Part model, mm, in its own coordinate system. Face numbers are marked on the shaded views. A direction names the side the tool comes from. Coordinates: 2 decimals unless noted, no trailing zeros. Order: outer loops, then holes, each group sorted by start corner. A loop starts at its lowest first (then second) coordinate and runs counter-clockwise, first axis right, second up.
```python
from build123d import *

# Parameters (mm, degrees)
SKETCH_1_R          = 11
EXTRUDE_1_DEPTH     = 2
SKETCH_2_R          = 5
EXTRUDE_2_DEPTH     = 10
SKETCH_4_R          = 3
CUT_EXTRUDE_2_DEPTH = 13
CUT_EXTRUDE_3_REACH = 4
SKETCH_5_R          = 1.5


with BuildPart() as part:
    # 草图1 → 凸台-拉伸1 (new body)
    with BuildSketch(Plane.XY):
        Circle(SKETCH_1_R)
    extrude(amount=EXTRUDE_1_DEPTH)

    # 草图2 → 凸台-拉伸2 (add)
    with BuildSketch(Plane.XY.offset(2)):
        Circle(SKETCH_2_R)
    extrude(amount=EXTRUDE_2_DEPTH)

    # 草图4 → 切除-拉伸2 (cut, through all)
    with BuildSketch(Plane.XY.offset(12)):
        Circle(SKETCH_4_R)
    extrude(amount=-CUT_EXTRUDE_2_DEPTH, mode=Mode.SUBTRACT)

    # 草图5 → 切除-拉伸3 (cut, up to next)
    with BuildSketch(Plane.XY.offset(2), mode=Mode.PRIVATE) as cut_extrude_3_sk1:
        with Locations((-8, 0)):
            Circle(SKETCH_5_R)
    cut_extrude_3_tool1 = extrude(cut_extrude_3_sk1.sketch, amount=-CUT_EXTRUDE_3_REACH, mode=Mode.PRIVATE) & part.part
    add(cut_extrude_3_tool1.solids().sort_by_distance((-8, 0, 2))[0], mode=Mode.SUBTRACT)
    # 草图5 → 切除-拉伸3 (cut, up to next)
    with BuildSketch(Plane.XY.offset(2), mode=Mode.PRIVATE) as cut_extrude_3_sk2:
        with Locations((0, 8)):
            Circle(SKETCH_5_R)
    cut_extrude_3_tool2 = extrude(cut_extrude_3_sk2.sketch, amount=-CUT_EXTRUDE_3_REACH, mode=Mode.PRIVATE) & part.part
    add(cut_extrude_3_tool2.solids().sort_by_distance((0, 8, 2))[0], mode=Mode.SUBTRACT)
    # 草图5 → 切除-拉伸3 (cut, up to next)
    with BuildSketch(Plane.XY.offset(2), mode=Mode.PRIVATE) as cut_extrude_3_sk3:
        with Locations((8, 0)):
            Circle(SKETCH_5_R)
    cut_extrude_3_tool3 = extrude(cut_extrude_3_sk3.sketch, amount=-CUT_EXTRUDE_3_REACH, mode=Mode.PRIVATE) & part.part
    add(cut_extrude_3_tool3.solids().sort_by_distance((8, 0, 2))[0], mode=Mode.SUBTRACT)
    # 草图5 → 切除-拉伸3 (cut, up to next)
    with BuildSketch(Plane.XY.offset(2), mode=Mode.PRIVATE) as cut_extrude_3_sk4:
        with Locations((0, -8)):
            Circle(SKETCH_5_R)
    cut_extrude_3_tool4 = extrude(cut_extrude_3_sk4.sketch, amount=-CUT_EXTRUDE_3_REACH, mode=Mode.PRIVATE) & part.part
    add(cut_extrude_3_tool4.solids().sort_by_distance((0, -8, 2))[0], mode=Mode.SUBTRACT)


solid = part.part
```
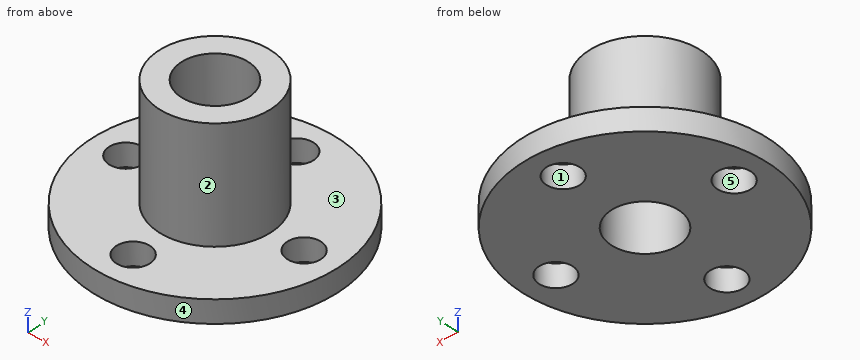
(1) Pull direction X, two halves, no side cores. Call the marked faces 3, 4 and 5: +X half, -X half, draft (parallel to the pull), parting line (faces both ways), or undercut.
(2) Slice it at C-C, the plane y = -8.75. Give the cut face in (x, z), then the cut area to 3 significant figures.
(3) Slice it at A-A, the plane y = 0. Give the cut face in (x, z), then the cut area to 3 significant figures.
(4) Probe line 1 (Y direction, x = 0, z = 0.5); line 2 (Z direction, x = 5, y = -8.5); line 3 (Y direction, x = -1.25, z = 1.25). List the from-to ranges inside material, lowest first.
(5) Tool access for the marked faces 1 and 2: list every direction of +Z, -Z, +X, -X, +Y, -Y with a clear straight run to the whole face (end or side of a thin tool).
(6) Drop flat-ended pins along their axis: pin 1 (5 mm diameter, centred on y = 5.5, z = 6, fed in from -X); pin 2 (1.5 mm diameter, centred on y = 1.5, z = 3, fed in from -X); pin 3 (3.5 mm diameter, centred on x = 0, y = -8, fed in from +Z). Give the stop position or say it passes through.
(7) Slice it at D-D, the plane x = -8. Give the cut face in (y, z).
Here are the results:
1. face 3: draft
1. face 4: parting line
1. face 5: undercut
2. outline: (-6.67, 0) - (-1.3, 0) - (-1.3, 2) - (-6.67, 2) - close; (1.3, 0) - (6.67, 0) - (6.67, 2) - (1.3, 2) - close
2. area: 21.5 mm2
3. outline: (-11, 0) - (-9.5, 0) - (-9.5, 2) - (-11, 2) - close; (-6.5, 0) - (-3, 0) - (-3, 12) - (-5, 12) - (-5, 2) - (-6.5, 2) - close; (3, 0) - (6.5, 0) - (6.5, 2) - (5, 2) - (5, 12) - (3, 12) - close; (9.5, 0) - (11, 0) - (11, 2) - (9.5, 2) - close
3. area: 60.0 mm2
4. line 1: y = -11 to -9.5, -6.5 to -3, 3 to 6.5, 9.5 to 11
4. line 2: z = 0 to 2
4. line 3: y = -10.93 to -8.83, -7.17 to -2.73, 2.73 to 7.17, 8.83 to 10.93
5. face 1: +Z, -Z
5. face 2: +Z
6. pin 1: stops at x = -4
6. pin 2: stops at x = -4.94
6. pin 3: stops at z = 2
7. outline: (-7.55, 0) - (-1.5, 0) - (-1.5, 2) - (-7.55, 2) - close; (1.5, 0) - (7.55, 0) - (7.55, 2) - (1.5, 2) - close
